```python
from build123d import *

# Parameters (mm, degrees)
SKETCH_1_W          = 8
SKETCH_1_H          = 22
EXTRUDE_1_DEPTH     = 10
SKETCH_1_3_W        = 8
SKETCH_1_3_H        = 22
EXTRUDE_2_DEPTH     = 30
EXTRUDE_3_DEPTH     = 4
SKETCH_3_R          = 6
CUT_EXTRUDE_1_DEPTH = 5
SKETCH_4_R          = 3
CUT_EXTRUDE_2_DEPTH = 31.618621785
SKETCH_5_R          = 5.5
CUT_EXTRUDE_3_DEPTH = 50.623583103
SKETCH_6_W          = 50
SKETCH_6_H          = 10
CUT_EXTRUDE_4_DEPTH = 3


with BuildPart() as part:
    # Эскиз1 → Бобышка-Вытянуть1 (new body)
    with BuildSketch(Plane.XY):
        Polygon((-12.5, -9.5), (-12.5, -12.5), (12.5, -12.5), (12.5, 12.5), (-4.5, 12.5), (-4.5, -9.5), align=None)
        with Locations((-8.5, 1.5)):
            Rectangle(SKETCH_1_W, SKETCH_1_H)
    extrude_1 = extrude(amount=EXTRUDE_1_DEPTH)

    # Эскиз1<3> → Бобышка-Вытянуть2 (add)
    with BuildSketch(Plane.XY):
        with Locations((-8.5, 1.5)):
            Rectangle(SKETCH_1_3_W, SKETCH_1_3_H)
    extrude_2 = extrude(amount=EXTRUDE_2_DEPTH)

    # Эскиз2 → Бобышка-Вытянуть3 (add)
    with BuildSketch(Plane(origin=(0, 12.5, 0), x_dir=(1, 0, 0), z_dir=(0, 1, 0))):
        Polygon((12.5, -10), (-4.5, -30), (-4.5, -10), align=None)
    extrude_3 = extrude(amount=-EXTRUDE_3_DEPTH)

    # Эскиз3 → Вырез-Вытянуть1 (cut)
    with BuildSketch(Plane.XY.offset(10)):
        with Locations((5.5, 1.5)):
            Circle(SKETCH_3_R)
    cut_extrude_1 = extrude(amount=-CUT_EXTRUDE_1_DEPTH, mode=Mode.SUBTRACT)

    # Эскиз4 → Вырез-Вытянуть2 (cut, through all)
    with BuildSketch(Plane.XY.offset(5)):
        with Locations((5.5, 1.5)):
            Circle(SKETCH_4_R)
    cut_extrude_2 = extrude(amount=-CUT_EXTRUDE_2_DEPTH, mode=Mode.SUBTRACT)

    # Зеркальное отражение1: Бобышка-Вытянуть1, Бобышка-Вытянуть2, Бобышка-Вытянуть3, Вырез-Вытянуть1, Вырез-Вытянуть2 across plane
    add(extrude_1.mirror(Plane(origin=(-12.5, 0, 10), x_dir=(0, 0, 1), z_dir=(-1, 0, 0))))
    add(extrude_2.mirror(Plane(origin=(-12.5, 0, 10), x_dir=(0, 0, 1), z_dir=(-1, 0, 0))))
    add(extrude_3.mirror(Plane(origin=(-12.5, 0, 10), x_dir=(0, 0, 1), z_dir=(-1, 0, 0))))
    add(cut_extrude_1.mirror(Plane(origin=(-12.5, 0, 10), x_dir=(0, 0, 1), z_dir=(-1, 0, 0))), mode=Mode.SUBTRACT)
    add(cut_extrude_2.mirror(Plane(origin=(-12.5, 0, 10), x_dir=(0, 0, 1), z_dir=(-1, 0, 0))), mode=Mode.SUBTRACT)

    # Эскиз5 → Вырез-Вытянуть3 (cut, through all)
    with BuildSketch(Plane.XY.offset(30)):
        with Locations((-12.5, 1.5)):
            Circle(SKETCH_5_R)
    extrude(amount=-CUT_EXTRUDE_3_DEPTH, mode=Mode.SUBTRACT)

    # Эскиз6 → Вырез-Вытянуть4 (cut)
    with BuildSketch(Plane.XZ.offset(12.5)):
        with Locations((-12.5, 5)):
            Rectangle(SKETCH_6_W, SKETCH_6_H)
    extrude(amount=-CUT_EXTRUDE_4_DEPTH, mode=Mode.SUBTRACT)


solid = part.part
```
Here's how the part is built. I have some questions about the finished solid (model axes, mm). A direction names the side the tool comes from. Coordinates: 2 decimals unless noted, no trailing zeros. Loops run counter-clockwise (first coordinate to the right, second up) from the corner with the lowest first, then second, coordinate; pieces in that order, holes last. Notation, with made-up numbers: (37, 80) - (86, 80) arc R8 ccw to (86, 93) - close; hole circle Ø2 at (45.25, -0.75). An arc over 180 degrees is marked (long way). Return JSON: item names as keys, results as strings. Group by question number.
Item 1: If we section it at A-A on x = -12.5: Write out the boundary of the cut face in (y, z).
Item 2: I need wall thicknesses on line 1 (Y direction, x = -30.5, z = 1.3); line 2 (Y direction, x = -12.5, z = 18.5); line 3 (X direction, y = 1, z = 8). Which ranges of each line are inside material? Lowest first, please. Write a range as from..to.
Item 3: We'd pull the mould along Y, two halves only. Please class faces 1 (the face through (8.27, 0.35, 2.54)), 2 (the face through (0, 8.5, 15)), 3 (the face through (0, -2, 10)): +Y half, -Y half, draft (parallel to the pull), parting line (faces both ways), or undercut.
Item 4: If we section it at D-D on y = -3: Write out the boundary of the cut face in (x, z).
Item 5: If we section it at C-C on z = 5.75: Write out the boundary of the cut face in (x, y), and give its area (3 significant figures).
Item 6: Will these pins go through, and if not, where does the flat tip stop? P1, Ø6, axis at x = -31.5, y = -4, coming from the +Z side; P2, Ø1, axis at y = 0.5, z = 21.5, coming from the -X side; P3, Ø7, axis at x = 5.5, y = 1.5, coming from the -Z side; P4, Ø7, axis at x = -30.5, y = 1.5, coming from the +Z side.
Item 7: If we section it at B-B on y = 8: Write out the boundary of the cut face in (x, z).
Item 8: On a 3-axis mill with a long thin cutter (end or side, diameter ignored), from which of +Z, -Z, +X, -X, +Y, -Y can I reach the whole of each face in a straight line? I mean faces 4 (the face through (-33, -1, 5)), 5 (the face through (-4.5, -1, 20)), 6 (the face through (-20.5, -1, 20)). Say none if no direction works.
Calculated:
{
 "1": {"outline": "(-9.5, 0) - (-4, 0) - (-4, 30) - (-9.5, 30) - close; (7, 0) - (12.5, 0) - (12.5, 30) - (7, 30) - close"},
 "2": {"line 1": "y = -9.5..-1.5, 4.5..12.5", "line 2": "y = -9.5..-4, 7..12.5", "line 3": "x = -37.5..-36.48, -24.52..-17.98, -7.02..-0.48, 11.48..12.5"},
 "3": {"face 1": "undercut", "face 2": "-Y half", "face 3": "draft"},
 "4": {"outline": "(-37.5, 0) - (-15.66, 0) - (-15.66, 30) - (-20.5, 30) - (-20.5, 10) - (-26.53, 10) - (-26.53, 5) - (-34.47, 5) - (-34.47, 10) - (-37.5, 10) - close; (-9.34, 0) - (12.5, 0) - (12.5, 10) - (9.47, 10) - (9.47, 5) - (1.53, 5) - (1.53, 10) - (-4.5, 10) - (-4.5, 30) - (-9.34, 30) - close"},
 "5": {"outline": "(-37.5, -9.5) - (12.5, -9.5) - (12.5, 12.5) - (-37.5, 12.5) - close; hole circle Ø12 at (-30.5, 1.5); hole circle Ø11 at (-12.5, 1.5); hole circle Ø12 at (5.5, 1.5)", "area": "779 mm^2"},
 "6": {"P1": "stops at z = 10", "P2": "stops at x = -20.5", "P3": "stops at z = 0", "P4": "stops at z = 5"},
 "7": {"outline": "(-37.5, 0) - (12.5, 0) - (12.5, 10) - (-4.5, 10) - (-4.5, 30) - (-20.5, 30) - (-20.5, 10) - (-37.5, 10) - close"},
 "8": {"face 4": "+Z", "face 5": "+Z, +X, -Y", "face 6": "+Z, -X, -Y"}
}
